Verification items for the finished model (mm, model axes). Face numbers are marked on the shaded views. A direction names the side the tool comes from. Coordinates: 2 decimals unless noted, no trailing zeros. Order: outer loops, then holes, each group sorted by start corner. A loop starts at its lowest first (then second) coordinate and runs counter-clockwise, first axis right, second up. Notation, with made-up numbers: (69, 85) -> (88, 85) arc R19 ccw to (88, 113) -> close; hole circle Ø1 at (73, 35). An arc over 180 degrees is marked (long way). Write item = value, one per line. Start each with the question number.
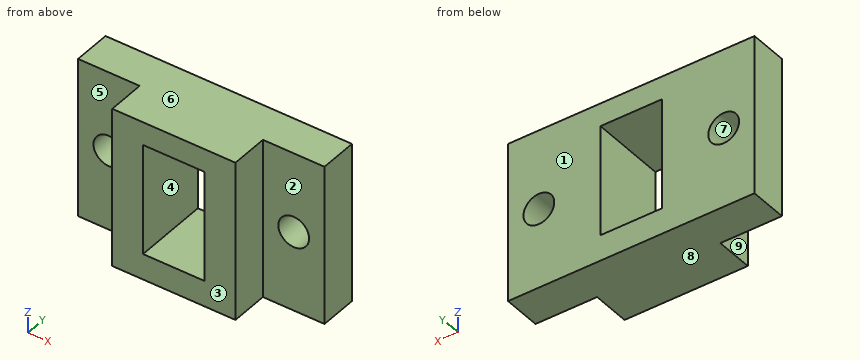
from build123d import *

# Parameters (mm, degrees)
SKETCH1_W           = 25.4
SKETCH1_H           = 15.621
BOSS_EXTRUDE1_DEPTH = 12.7
SKETCH4_W           = 6.35
SKETCH4_H           = 15.621
BOSS_EXTRUDE4_DEPTH = 22.86
SKETCH5_W           = 25.4
SKETCH5_H           = 7.9375
CUT_EXTRUDE1_DEPTH  = 15.748
SKETCH6_W           = 25.4
SKETCH6_H           = 15.621
BOSS_EXTRUDE5_DEPTH = 5.334
SKETCH7_W           = 32.9565
SKETCH7_H           = 7.8105
BOSS_EXTRUDE6_DEPTH = 12.7
SKETCH8_W           = 32.9565
SKETCH8_H           = 7.8105
BOSS_EXTRUDE7_DEPTH = 12.7
SKETCH9_R           = 3.175
CUT_EXTRUDE2_DEPTH  = 12.7


with BuildPart() as part:
    # Sketch1 → Boss-Extrude1 (new body)
    with BuildSketch(Plane.XY):
        Rectangle(SKETCH1_W, SKETCH1_H)
    extrude(amount=BOSS_EXTRUDE1_DEPTH)

    # Sketch4 → Boss-Extrude4 (add)
    with BuildSketch(Plane(origin=(0, 0, 0), x_dir=(-1, 0, 0), z_dir=(0, 0, -1))):
        with Locations((9.525, 0)):
            Rectangle(SKETCH4_W, SKETCH4_H)
        with Locations((-9.525, 0)):
            Rectangle(SKETCH4_W, SKETCH4_H)
    extrude(amount=BOSS_EXTRUDE4_DEPTH)

    # Sketch5 → Cut-Extrude1 (cut)
    with BuildSketch(Plane(origin=(0, 7.8105, 0), x_dir=(1, 0, 0), z_dir=(0, 1, 0))):
        with Locations((0, -8.73125)):
            Rectangle(SKETCH5_W, SKETCH5_H)
    extrude(amount=-CUT_EXTRUDE1_DEPTH, mode=Mode.SUBTRACT)

    # Sketch6 → Boss-Extrude5 (add)
    with BuildSketch(Plane(origin=(0, 0, -22.86), x_dir=(-1, 0, 0), z_dir=(0, 0, -1))):
        Rectangle(SKETCH6_W, SKETCH6_H)
    extrude(amount=BOSS_EXTRUDE5_DEPTH)

    # Sketch7 → Boss-Extrude6 (add)
    with BuildSketch(Plane.ZY.offset(12.7)):
        with Locations((-11.71575, 3.90525)):
            Rectangle(SKETCH7_W, SKETCH7_H)
    extrude(amount=BOSS_EXTRUDE6_DEPTH)

    # Sketch8 → Boss-Extrude7 (add)
    with BuildSketch(Plane(origin=(12.7, 0, 0), x_dir=(0, 0, -1), z_dir=(1, 0, 0))):
        with Locations((11.71575, 3.90525)):
            Rectangle(SKETCH8_W, SKETCH8_H)
    extrude(amount=BOSS_EXTRUDE7_DEPTH)

    # Sketch9 → Cut-Extrude2 (cut)
    with BuildSketch(Plane.XZ):
        with Locations((-19.05, -11.71575)):
            Circle(SKETCH9_R)
        with Locations((19.05, -11.71575)):
            Circle(SKETCH9_R)
    extrude(amount=-CUT_EXTRUDE2_DEPTH, mode=Mode.SUBTRACT)


solid = part.part
Item 1: Section check D-D (y = 2.25). State how many separate pieces and enclosed holes the cut face has, then the cut area to 3 significant figures.
Item 2: Section check C-C (x = -19.05). Record the boundary of the cut face in (y, z), then the cut area to 3 significant figures.
Item 3: Gauge pin test, flat ends, axial feed: P1, Ø6.5, axis at x = 22, z = -15.5, coming from the -Y side; P2, Ø2, axis at x = 16, y = -2.5, coming from the +Z side; P3, Ø4, axis at y = -5.5, z = -16, coming from the +X side; P4, Ø6, axis at y = -5.5, z = -20, coming from the -X side. Record the tip position at first contact, or that the pin passes through.
Item 4: Section check A-A (x = -4.5). Record the boundary of the cut face in (y, z).
Item 5: Thickness scan on line 1 (Z direction, x = -19.05, y = 3.5); line 2 (Z direction, x = 0, y = -6.75); line 3 (X direction, y = -6.25, z = -3.5). Record the ranges inside material, lowest first.
Item 6: Tool access check on the marked faces 1, 2, 3, 4 and 5. Record the directions out of +Z, -Z, +X, -X, +Y, -Y that give a thin tool (end or side, any length) a straight path to the whole face; none if there is none.
Item 7: Section check B-B (y = -2.5). Record the boundary of the cut face in (x, z), then the cut area to 3 significant figures.
Item 8: Mould release check, pull along Z, two halves, no side actions. Record for the marked faces 6, 7, 8 and 9: pulls with the +Z half, pulls with the -Z half, needs draft (parallel to the pull), parting line crosses it, or undercut.
Filled sheet:
q1.separate_pieces = 1
q1.enclosed_holes = 3
q1.area = 1,320 mm^2
q2.outline = (0, -28.19) -> (7.81, -28.19) -> (7.81, -14.89) -> (0, -14.89) -> close; (0, -8.54) -> (7.81, -8.54) -> (7.81, 4.76) -> (0, 4.76) -> close
q2.area = 208 mm^2
q3.P1 = 0
q3.P2 = through
q3.P3 = 12.7
q3.P4 = -12.7
q4.outline = (-7.81, -28.19) -> (7.81, -28.19) -> (7.81, -22.86) -> (-7.81, -22.86) -> close; (-7.81, 0) -> (7.81, 0) -> (7.81, 4.76) -> (-7.81, 4.76) -> close
q5.line_1 = -28.19 to -14.89, -8.54 to 4.76
q5.line_2 = -28.19 to -22.86, 0 to 4.76
q5.line_3 = -12.7 to -6.35, 6.35 to 12.7
q6.face_1 = +Z, -Z, +X, -X, +Y
q6.face_2 = +Z, -Z, +X, -Y
q6.face_3 = +Z, -Z, +X, -X, -Y
q6.face_4 = +Y, -Y
q6.face_5 = +Z, -Z, -X, -Y
q7.outline = (-12.7, -28.19) -> (12.7, -28.19) -> (12.7, 4.76) -> (-12.7, 4.76) -> close; hole (-6.35, -22.86) -> (6.35, -22.86) -> (6.35, 0) -> (-6.35, 0) -> close
q7.area = 547 mm^2
q8.face_6 = pulls with the +Z half
q8.face_7 = undercut
q8.face_8 = pulls with the -Z half
q8.face_9 = needs draft
